Answer from the drawing. Dimensions are ordinates in mm from the lowest x, y and z of the part. A direction names the side the tool comes from. Give positions to 0.01 mm unless a question says otherwise; leave off trailing zeros. Loops run counter-clockwise (first coordinate to the right, second up) from the corner with the lowest first, then second, coordinate; pieces in that order, holes last. Notation, with made-up numbers: M 56,37.5 L 81,37.5 A20 cw 81,47.5 Z; hole C -8.5,38.5 d1. An arc over 180 degrees is marked long. Use a Markdown table: item, result.
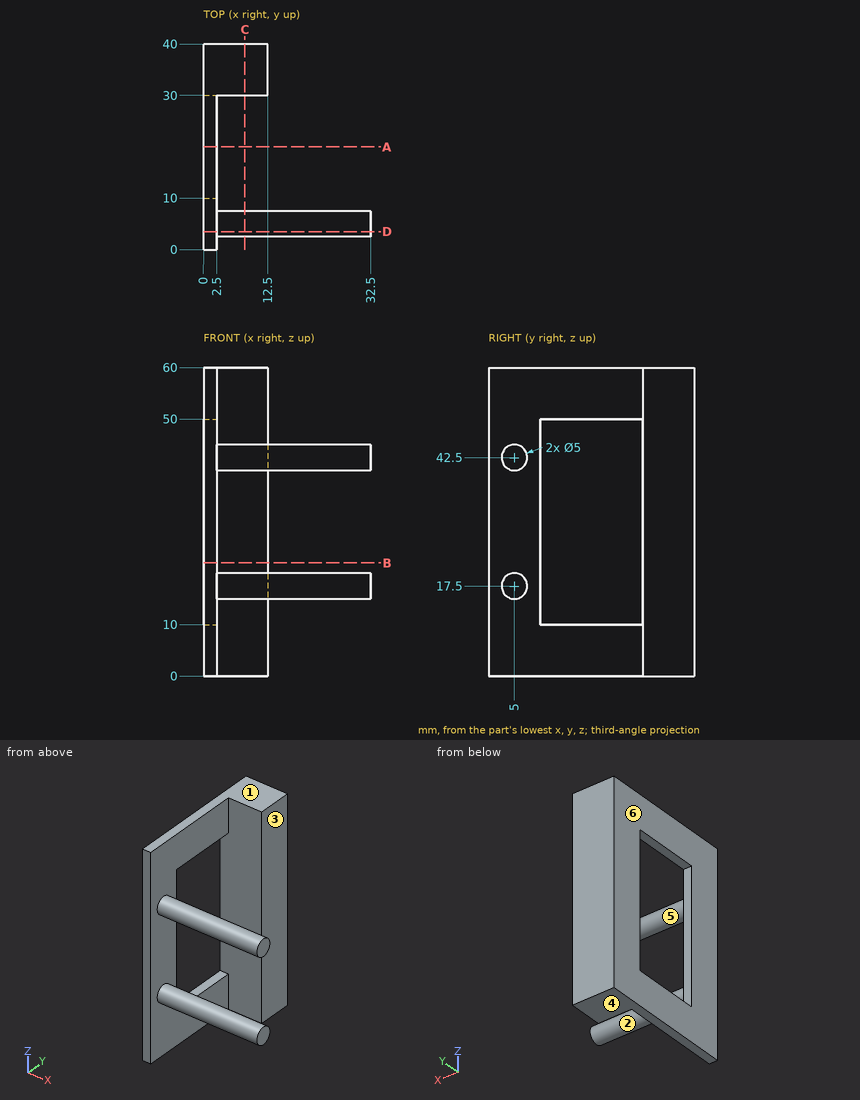
(1) The mould has two halves that part along Z. Classify the marked faces 4, 5 and 6: released by +Z, released by -Z, zero draft, split by the parting line, or undercut.
Entries:
| item | result |
|---|---|
| face 4 | released by -Z |
| face 5 | undercut |
| face 6 | zero draft |
(2) Which of the six approach directions +Z, -Z, +X, -X, +Y, -Y give full straight-line access (tool end or side, diameter ignored) to the marked faces 1, 2 and 3?
Entries:
| item | result |
|---|---|
| face 1 | +Z, +X, -X, +Y, -Y |
| face 2 | +X |
| face 3 | +Z, -Z, +X, +Y |
(3) Given P1, Ø3, axis at y = 14, z = 47, coming from the +X side; P2, Ø15, axis at y = 17, z = 40.5, coming from the +X side; P3, Ø5, axis at y = 36, z = 18.5, coming from the +X side; P4, Ø10, axis at x = 9, z = 42.5, coming from the -Y side, each flat-ended and moving along its own axis, determine where each tip first touches the part or whether it passes through.
Entries:
| item | result |
|---|---|
| P1 | passes through |
| P2 | stops at x = 2.5 |
| P3 | stops at x = 12.5 |
| P4 | stops at y = 2.5 |
(4) Consider probe 1 along Z at (x, y) = (2, 21.5); probe 2 along X at (y, z) = (37, 29.5); probe 3 along X at (y, z) = (16, 8). Determine where each line is inside the solid, lowest interval first. Write a range as [from, to].
Entries:
| item | result |
|---|---|
| probe 1 | z = [0, 10], [50, 60] |
| probe 2 | x = [0, 12.5] |
| probe 3 | x = [0, 2.5] |
(5) A cutting plane is placed at D-D (y = 3.5). Write down the section's boundary in (x, z).
Entries:
| item | result |
|---|---|
| outline | M 0,0 L 2.5,0 L 2.5,15.5 L 32.5,15.5 L 32.5,19.5 L 2.5,19.5 L 2.5,40.5 L 32.5,40.5 L 32.5,44.5 L 2.5,44.5 L 2.5,60 L 0,60 Z |
(6) A cutting plane is placed at A-A (y = 20). Write down the section's boundary in (x, z).
Entries:
| item | result |
|---|---|
| outline | M 0,0 L 2.5,0 L 2.5,10 L 0,10 Z; M 0,50 L 2.5,50 L 2.5,60 L 0,60 Z |
(7) A cutting plane is placed at C-C (x = 8). Write down the section's boundary in (y, z).
Entries:
| item | result |
|---|---|
| outline | C 5,17.5 d5; C 5,42.5 d5; M 30,0 L 40,0 L 40,60 L 30,60 Z |
(8) A cutting plane is placed at B-B (z = 22). Write down the section's boundary in (x, y).
Entries:
| item | result |
|---|---|
| outline | M 0,0 L 2.5,0 L 2.5,10 L 0,10 Z; M 0,30 L 12.5,30 L 12.5,40 L 0,40 Z |
